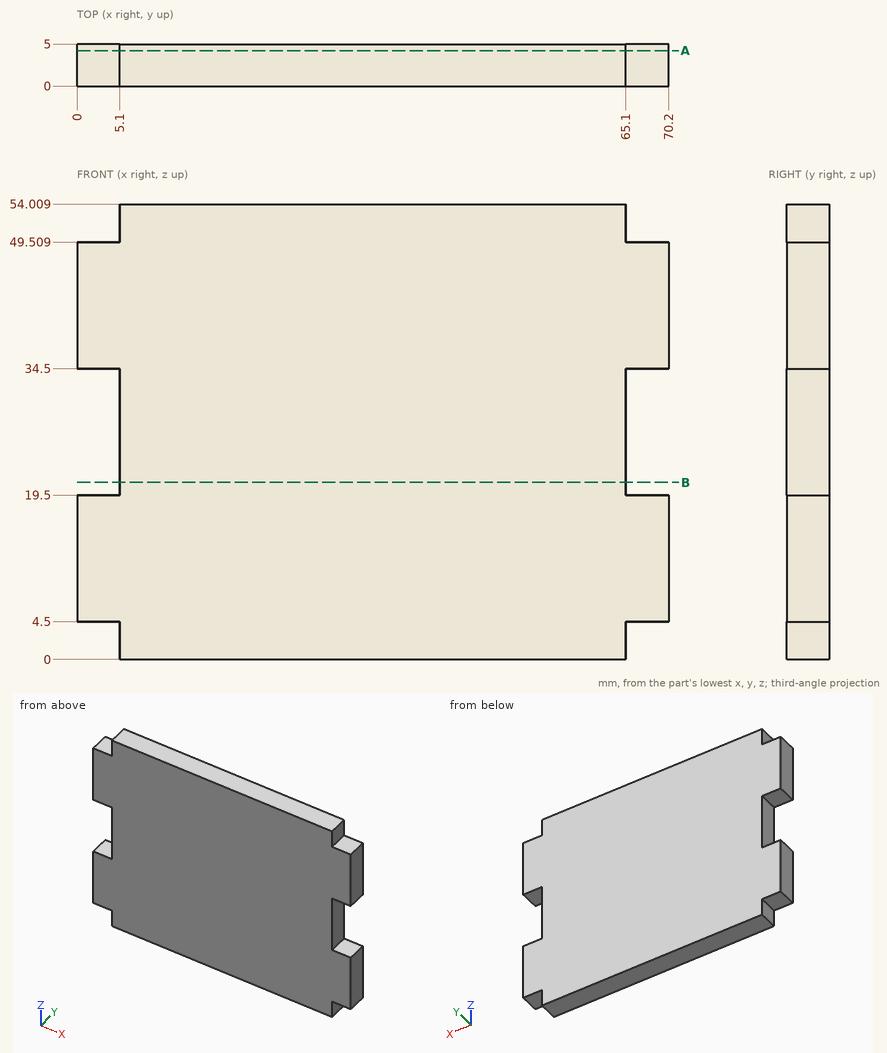
The drawing under review shows one solid part. Ordinate dimensions are in mm from its lowest x, y, z. Round coordinates to 2 decimals unless told otherwise and drop trailing zeros. Loops run counter-clockwise (first coordinate to the right, second up) from the corner with the lowest first, then second, coordinate; pieces in that order, holes last. Notation, with made-up numbers: (1, 30) - (51, 30) arc R30 cw to (51, 66) - close; hole circle Ø6 at (69, -20.5). An arc over 180 degrees is marked (long way). Use one line per item in the form item = value.
Item 1: For line 1 (X direction, y = 2.65, z = 50); line 2 (Z direction, x = 65.5, y = 3.25), list the stretches that pass through material, from the lowest coordinate up.
Answers:
line_1 = 5.1 to 65.1
line_2 = 4.5 to 19.5, 34.5 to 49.51
Item 2: Consider section A-A on y = 4.2. Write out the cut boundary in (x, z).
Answers:
outline = (0, 4.5) - (5.1, 4.5) - (5.1, 0) - (65.1, 0) - (65.1, 4.5) - (70.2, 4.5) - (70.2, 19.5) - (65.1, 19.5) - (65.1, 34.5) - (70.2, 34.5) - (70.2, 49.51) - (65.1, 49.51) - (65.1, 54.01) - (5.1, 54.01) - (5.1, 49.51) - (0, 49.51) - (0, 34.5) - (5.1, 34.5) - (5.1, 19.5) - (0, 19.5) - close
Item 3: Consider section B-B on z = 21. Write out the cut boundary in (x, y).
Answers:
outline = (5.1, 0) - (65.1, 0) - (65.1, 5) - (5.1, 5) - close
Item 4: Clearance check with flat-ended pins moving along their axes: P1, Ø2.5, axis at x = 2, y = 2, coming from the +Z side; P2, Ø1.3, axis at y = 3, z = 51, coming from the -X side; P3, Ø2.5, axis at x = 2.5, y = 3.5, coming from the -Z side. State where each tip first meets the part, or that it passes through.
Answers:
P1 = 49.51
P2 = 5.1
P3 = 4.5
